For this review, take the finished solid that the model builds, in its own axes (mm). A direction names the side the tool comes from. Give positions to 0.01 mm unless a question says otherwise; leave off trailing zeros. Order: outer loops, then holes, each group sorted by start corner. A loop starts at its lowest first (then second) coordinate and runs counter-clockwise, first axis right, second up. Notation, with made-up numbers: (82.25, 8) -> (140.25, 8) arc R19 ccw to (140.25, 12) -> close; hole circle Ø9 at (12, 22.5). An arc over 180 degrees is marked (long way). Return JSON: item names as keys, results as strings. Group by question number.
1) The part is to be moulded in two halves that separate along X. For faces 3 (the face through (40, 2, 20)), 4 (the face through (20, 2.3, 24)), 5 (the face through (20, 5, 20)), say which applies: released by +X, released by -X, zero draft, split by the parting line, or undercut.
2) For faces 1 (the face through (20, 2, 40)), 2 (the face through (21.983, 3.669, 17.24)), list the 3-axis set-ups (+Z, -Z, +X, -X, +Y, -Y) from which the entire face can be reached by the end or side of a thin tool; tool diameter is ignored.
3) To check wall thickness, follow line 1 along X through (y, z) = (1.15, 17.5); line 2 along X through (y, z) = (2.9, 17.5). State the ranges of each line that lie inside material, in increasing order.
4) Add section A-A (z = 22.5). Give the boundary of the cut face in (x, y).
5) Insertion check: P1, Ø3.5, axis at x = 20, z = 22.5, coming from the +Y side. The pin has a flat end and moves straight along its axis. Give the tip position at first contact, or say it passes through.
6) Add section B-B (x = 20). Give the boundary of the cut face in (y, z).
from build123d import *

# Parameters (mm, degrees)
SKETCH_1_W          = 40
SKETCH_1_H          = 40
EXTRUDE_1_DEPTH     = 5
SKETCH_2_R          = 1.2
CUT_EXTRUDE_1_DEPTH = 57.789083458
SKETCH_3_R          = 2
CUT_EXTRUDE_2_DEPTH = 2.7


with BuildPart() as part:
    # 草图1 → 凸台-拉伸1 (new body)
    with BuildSketch(Plane(origin=(0, 0, 0), x_dir=(1, 0, 0), z_dir=(0, 1, 0))):
        with Locations((20, -20)):
            Rectangle(SKETCH_1_W, SKETCH_1_H)
    extrude(amount=EXTRUDE_1_DEPTH)

    # 草图2 → 切除-拉伸1 (cut, through all)
    with BuildSketch(Plane(origin=(0, 5, 0), x_dir=(1, 0, 0), z_dir=(0, 1, 0))):
        with Locations(Location((20, -17.5, 0), (0, 0, 270))):
            Circle(SKETCH_2_R)
        with Locations(Location((20, -22.5, 0), (0, 0, 270))):
            Circle(SKETCH_2_R)
    extrude(amount=-CUT_EXTRUDE_1_DEPTH, mode=Mode.SUBTRACT)

    # 草图3 → 切除-拉伸2 (cut)
    with BuildSketch(Plane(origin=(0, 5, 0), x_dir=(1, 0, 0), z_dir=(0, 1, 0))):
        with Locations(Location((20, -17.5, 0), (0, 0, 270))):
            Circle(SKETCH_3_R)
        with Locations(Location((20, -22.5, 0), (0, 0, 270))):
            Circle(SKETCH_3_R)
    extrude(amount=-CUT_EXTRUDE_2_DEPTH, mode=Mode.SUBTRACT)


solid = part.part
Evaluation:
{
 "1": {"face 3": "released by +X", "face 4": "undercut", "face 5": "zero draft"},
 "2": {"face 1": "+Z, +X, -X, +Y, -Y", "face 2": "+Y"},
 "3": {"line 1": "0 to 18.8, 21.2 to 40", "line 2": "0 to 18, 22 to 40"},
 "4": {"outline": "(0, 0) -> (18.8, 0) -> (18.8, 2.3) -> (18, 2.3) -> (18, 5) -> (0, 5) -> close; (21.2, 0) -> (40, 0) -> (40, 5) -> (22, 5) -> (22, 2.3) -> (21.2, 2.3) -> close"},
 "5": {"P1": "y = 2.3"},
 "6": {"outline": "(0, 0) -> (5, 0) -> (5, 15.5) -> (2.3, 15.5) -> (2.3, 16.3) -> (0, 16.3) -> close; (0, 18.7) -> (2.3, 18.7) -> (2.3, 19.5) -> (5, 19.5) -> (5, 20.5) -> (2.3, 20.5) -> (2.3, 21.3) -> (0, 21.3) -> close; (0, 23.7) -> (2.3, 23.7) -> (2.3, 24.5) -> (5, 24.5) -> (5, 40) -> (0, 40) -> close"}
}
